from build123d import *

# Parameters (mm, degrees)
SKETCH_1_R          = 11
SKETCH_1_R_2        = 1.75
EXTRUDE_1_DEPTH     = 5
SKETCH_2_R          = 4
SKETCH_2_R_2        = 2.35
CUT_EXTRUDE_1_DEPTH = 10


with BuildPart() as part:
    # 스케치1 → 보스-돌출1 (new body)
    with BuildSketch(Plane.XY):
        Circle(SKETCH_1_R)
        with Locations((0, 8)):
            Circle(SKETCH_1_R_2, mode=Mode.SUBTRACT)
        with Locations((8, 0)):
            Circle(SKETCH_1_R_2, mode=Mode.SUBTRACT)
        with Locations((0, -8)):
            Circle(SKETCH_1_R_2, mode=Mode.SUBTRACT)
        with Locations((-8, 0)):
            Circle(SKETCH_1_R_2, mode=Mode.SUBTRACT)
    extrude(amount=EXTRUDE_1_DEPTH)

    # 스케치2 → 컷-돌출1 (cut)
    # profile 1 of 2: a face of its own
    with BuildSketch(Plane.XY.offset(5)):
        Circle(SKETCH_2_R)
        Circle(SKETCH_2_R_2, mode=Mode.SUBTRACT)
    # profile 2 of 2: a face of its own
    with BuildSketch(Plane.XY.offset(5)):
        Circle(SKETCH_2_R_2)
    extrude(amount=-CUT_EXTRUDE_1_DEPTH, mode=Mode.SUBTRACT)


solid = part.part
For this review, take the finished solid that the model builds, in its own axes (mm). Round coordinates to 2 decimals unless told otherwise and drop trailing zeros. Write each loop counter-clockwise with the first axis right and the second up, starting at its lowest first coordinate (ties: lowest second). Pieces come first, ordered by that corner, then holes. Notation, with made-up numbers: (-7.75, 62.5) -> (0.25, 62.5) arc R30 ccw to (0.25, 90.5) -> close; hole circle Ø1 at (65, 5). An arc over 180 degrees is marked (long way). Put each result on its own line as item: value.
Q1. Clearance check with a flat-ended pin moving along its axis: pin 1 Ø2 at (x, y) = (8, 0) entering from +Z. State where the tip first meets the part, or that it passes through.
Determined:
pin 1: passes through
Q2. Consider section D-D on x = -1. State the section outline as (y, z) points, and give its area (3 significant figures).
Determined:
outline: (-10.95, 0) -> (-9.44, 0) -> (-9.44, 5) -> (-10.95, 5) -> close; (-6.56, 0) -> (-3.87, 0) -> (-3.87, 5) -> (-6.56, 5) -> close; (3.87, 0) -> (6.56, 0) -> (6.56, 5) -> (3.87, 5) -> close; (9.44, 0) -> (10.95, 0) -> (10.95, 5) -> (9.44, 5) -> close
area: 42.1 mm^2
Q3. Consider section C-C on z = 4.45. State the section outline as (x, y) points.
Determined:
outline: circle Ø22 at (0, 0); hole circle Ø3.5 at (-8, 0); hole circle Ø8 at (0, 0); hole circle Ø3.5 at (0, -8); hole circle Ø3.5 at (0, 8); hole circle Ø3.5 at (8, 0)
Q4. Consider section A-A on y = 0. State the section outline as (x, z) points.
Determined:
outline: (-11, 0) -> (-9.75, 0) -> (-9.75, 5) -> (-11, 5) -> close; (-6.25, 0) -> (-4, 0) -> (-4, 5) -> (-6.25, 5) -> close; (4, 0) -> (6.25, 0) -> (6.25, 5) -> (4, 5) -> close; (9.75, 0) -> (11, 0) -> (11, 5) -> (9.75, 5) -> close
Q5. Consider section B-B on x = -8. State the section outline as (y, z) points.
Determined:
outline: (-7.55, 0) -> (-1.75, 0) -> (-1.75, 5) -> (-7.55, 5) -> close; (1.75, 0) -> (7.55, 0) -> (7.55, 5) -> (1.75, 5) -> close
Q6. To check wall thickness, follow L1, parallel to Y at x = 0, z = 1.35; L2, parallel to Y at x = -1.5, z = 1.95; L3, parallel to X at y = 1.25, z = 2.7. State the ranges of each line that lie inside material, in increasing order. Write a range as [from, to].
Determined:
L1: y = [-11, -9.75], [-6.25, -4], [4, 6.25], [9.75, 11]
L2: y = [-10.9, -8.9], [-7.1, -3.71], [3.71, 7.1], [8.9, 10.9]
L3: x = [-10.93, -9.22], [-6.78, -3.8], [3.8, 6.78], [9.22, 10.93]
Q7. The part is to be moulded in two halves that separate along Y. For faces 1 (the cylindrical face through (-2.38, -10.74, 2.46)), 2 (the flat face through (0, -5, 0)), 3 (the cylindrical face through (-6.331, 0.526, 2.465)), say which applies: released by +Y, released by -Y, zero draft, split by the parting line, or undercut.
Determined:
face 1: split by the parting line
face 2: zero draft
face 3: undercut
